Part print with two shaded views. Sizes in mm from the minimum x, y, z corner. A direction names the side the tool comes from. Round coordinates to 2 decimals unless told otherwise and drop trailing zeros. Loops run counter-clockwise (first coordinate to the right, second up) from the corner with the lowest first, then second, coordinate; pieces in that order, holes last. Notation, with made-up numbers: (88, 54) - (110, 54) arc R21 ccw to (110, 72) - close; hole circle Ø11 at (43.25, 41). An arc over 180 degrees is marked (long way). Use a Markdown table: item, result.
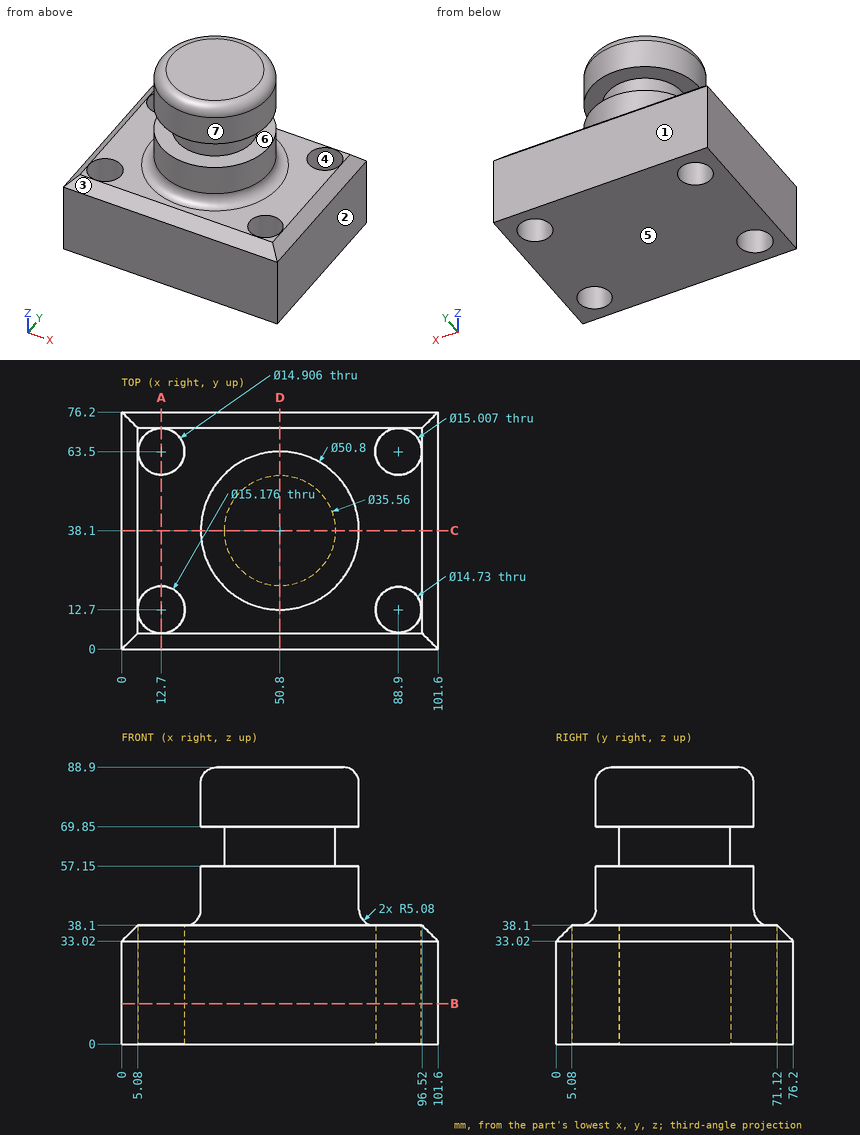
Q1. Pull direction Y, two halves, no side cores. Call the marked faces 1, 2, 3 and 4: pulls with the +Y half, pulls with the -Y half, needs draft (parallel to the pull), parting line crosses it, or undercut.
Results found:
| item | result |
|---|---|
| face 1 | pulls with the +Y half |
| face 2 | needs draft |
| face 3 | pulls with the -Y half |
| face 4 | undercut |
Q2. Probe line 1 (X direction, y = 63.5, z = 14); line 2 (X direction, y = 63, z = 28); line 3 (Y direction, x = 12.7, z = 12.5). List the from-to ranges inside material, lowest first.
Results found:
| item | result |
|---|---|
| line 1 | x = 0 to 5.25, 20.15 to 81.4, 96.4 to 101.6 |
| line 2 | x = 0 to 5.26, 20.14 to 81.41, 96.39 to 101.6 |
| line 3 | y = 0 to 5.11, 20.29 to 56.05, 70.95 to 76.2 |
Q3. Cut at D-D, the plane x = 50.8. List the corners of the cut face in (y, z), plus the area to 3 significant figures.
Results found:
| item | result |
|---|---|
| outline | (0, 0) - (76.2, 0) - (76.2, 33.02) - (71.12, 38.1) - (68.58, 38.1) arc R5.08 cw to (63.5, 43.18) - (63.5, 57.15) - (55.88, 57.15) - (55.88, 69.85) - (63.5, 69.85) - (63.5, 83.82) arc R5.08 ccw to (58.42, 88.9) - (17.78, 88.9) arc R5.08 ccw to (12.7, 83.82) - (12.7, 69.85) - (20.32, 69.85) - (20.32, 57.15) - (12.7, 57.15) - (12.7, 43.18) arc R5.08 cw to (7.62, 38.1) - (5.08, 38.1) - (0, 33.02) - close |
| area | 5,260 mm2 |
Q4. Cut at A-A, the plane x = 12.7. Count the separate pieces of the cut face and the enclosed holes in it, plus the area to 3 significant figures.
Results found:
| item | result |
|---|---|
| separate pieces | 3 |
| enclosed holes | 0 |
| area | 1,730 mm2 |
Q5. Which spindle directions (+Z, -Z, +X, -X, +Y, -Y) get a long thin tool onto all of the face, cutting with end or side? Do the marked faces 5, 6 and 7. Say none if no direction does.
Results found:
| item | result |
|---|---|
| face 5 | -Z, +X, -X, +Y, -Y |
| face 6 | none |
| face 7 | +Z |
Q6. Cut at C-C, the plane y = 38.1. List the corners of the cut face in (x, z), plus the area to 3 significant figures.
Results found:
| item | result |
|---|---|
| outline | (0, 0) - (101.6, 0) - (101.6, 33.02) - (96.52, 38.1) - (81.28, 38.1) arc R5.08 cw to (76.2, 43.18) - (76.2, 57.15) - (68.58, 57.15) - (68.58, 69.85) - (76.2, 69.85) - (76.2, 83.82) arc R5.08 ccw to (71.12, 88.9) - (30.48, 88.9) arc R5.08 ccw to (25.4, 83.82) - (25.4, 69.85) - (33.02, 69.85) - (33.02, 57.15) - (25.4, 57.15) - (25.4, 43.18) arc R5.08 cw to (20.32, 38.1) - (5.08, 38.1) - (0, 33.02) - close |
| area | 6,230 mm2 |
Q7. Drop flat-ended pins along their axis: pin 1 (9 mm diameter, centred on x = 88.9, y = 12.7, fed in from -Z); pin 2 (8 mm diameter, centred on y = 23.5, z = 56.5, fed in from -X); pin 3 (19.5 mm diameter, centred on x = 12.7, y = 63.5, fed in from +Z); pin 4 (3 mm diameter, centred on y = 19.5, z = 78.5, fed in from +X). Give the stop position or say it passes through.
Results found:
| item | result |
|---|---|
| pin 1 | passes through |
| pin 2 | stops at x = 27.72 |
| pin 3 | stops at z = 38.1 |
| pin 4 | stops at x = 69.58 |
Q8. Cut at B-B, the plane z = 13. List the corners of the cut face in (x, y) (1 decimal), plus the area to 3 significant figures.
Results found:
| item | result |
|---|---|
| outline | (0, 0) - (101.6, 0) - (101.6, 76.2) - (0, 76.2) - close; hole circle Ø15.2 at (12.7, 12.7); hole circle Ø14.9 at (12.7, 63.5); hole circle Ø15 at (88.9, 63.5); hole circle Ø14.7 at (88.9, 12.7) |
| area | 7,040 mm2 |
